```python
from build123d import *

# Parameters (mm, degrees)
SKIZZE1_W                       = 12
SKIZZE1_H                       = 17
AUFSATZ_LINEAR_AUSTRAGEN1_DEPTH = 2
SKIZZE3_W                       = 3
SKIZZE3_H                       = 1
SCHNITT_LINEAR_AUSTRAGEN1_DEPTH = 3
VERRUNDUNG1_R                   = 0.25


with BuildPart() as part:
    # Skizze1 → Aufsatz-Linear austragen1 (new body)
    with BuildSketch(Plane(origin=(0, 0, 0), x_dir=(1, 0, 0), z_dir=(0, 1, 0))):
        with Locations((6, 8.5)):
            Rectangle(SKIZZE1_W, SKIZZE1_H)
    extrude(amount=AUFSATZ_LINEAR_AUSTRAGEN1_DEPTH)

    # Skizze3 → Schnitt-Linear austragen1 (cut, through all)
    with BuildSketch(Plane(origin=(0, 2, 0), x_dir=(1, 0, 0), z_dir=(0, 1, 0))):
        with Locations((8.5, 2.5)):
            Rectangle(SKIZZE3_W, SKIZZE3_H)
        with Locations((3.5, 14.5)):
            Rectangle(SKIZZE3_W, SKIZZE3_H)
    extrude(amount=-SCHNITT_LINEAR_AUSTRAGEN1_DEPTH, mode=Mode.SUBTRACT)

    # Verrundung1
    verrundung1_edges = [part.edges().sort_by_distance(p)[0] for p in [
        (7, 1, -2),
        (10, 1, -2),
        (2, 1, -15),
        (5, 1, -15),
    ]]
    fillet(verrundung1_edges, radius=VERRUNDUNG1_R)


solid = part.part
```
Design review of the part built by this model. Coordinates are the model's own, in mm. A direction names the side the tool comes from. Coordinates: 2 decimals unless noted, no trailing zeros. Order: outer loops, then holes, each group sorted by start corner. A loop starts at its lowest first (then second) coordinate and runs counter-clockwise, first axis right, second up. Notation, with made-up numbers: (37.25, 19.25) - (72.25, 19.25) arc R25 cw to (72.25, 51.25) - close; hole circle Ø5 at (68.25, 18.25). An arc over 180 degrees is marked (long way). Answer in a Markdown table with one row per item.
(1) Clearance check with a flat-ended pin moving along its axis: pin 1 (1 mm diameter, centred on x = 3.5, y = 0.5, fed in from +Z). State where the tip first meets the part, or that it passes through.
Checked values:
| item | result |
|---|---|
| pin 1 | z = 0 |
(2) Consider section B-B on x = 9.5. State the section outline as (y, z) points, plus the area to 3 significant figures.
Checked values:
| item | result |
|---|---|
| outline | (0, -17) - (2, -17) - (2, -3) - (0, -3) - close; (0, -2) - (2, -2) - (2, 0) - (0, 0) - close |
| area | 32.0 mm^2 |
(3) The part is to be moulded in two halves that separate along X. For faces 3 (the flat face through (3, 1, -14)), 4 (the flat face through (6, 1, -17)), 5 (the flat face through (3, 1, -15)), 6 (the flat face through (0, 1, -8)), say which applies: released by +X, released by -X, zero draft, split by the parting line, or undercut.
Checked values:
| item | result |
|---|---|
| face 3 | undercut |
| face 4 | zero draft |
| face 5 | undercut |
| face 6 | released by -X |
(4) Consider section C-C on y = 0.2. State the section outline as (x, z) points.
Checked values:
| item | result |
|---|---|
| outline | (0, -17) - (12, -17) - (12, 0) - (0, 0) - close; hole (2, -14.75) arc R0.25 ccw to (2.25, -15) - (4.75, -15) arc R0.25 ccw to (5, -14.75) - (5, -14) - (2, -14) - close; hole (7, -3) - (10, -3) - (10, -2.25) arc R0.25 ccw to (9.75, -2) - (7.25, -2) arc R0.25 ccw to (7, -2.25) - close |
(5) Consider section A-A on z = -2.5. State the section outline as (x, y) points, plus the area to 3 significant figures.
Checked values:
| item | result |
|---|---|
| outline | (0, 0) - (7, 0) - (7, 2) - (0, 2) - close; (10, 0) - (12, 0) - (12, 2) - (10, 2) - close |
| area | 18.0 mm^2 |
(6) For faces 1 (the flat face through (6, 1, 0)), 2 (the flat face through (8, 1, -3)), list the 3-axis set-ups (+Z, -Z, +X, -X, +Y, -Y) from which the entire face can be reached by the end or side of a thin tool; tool diameter is ignored.
Checked values:
| item | result |
|---|---|
| face 1 | +Z, +X, -X, +Y, -Y |
| face 2 | +Y, -Y |
(7) Wall thickness on line 1 along Z through (x, y) = (3.75, 0.2); line 2 along Z through (x, y) = (8.75, 1): over which ranges is each line inside the solid? List them lowest first. Write a range as from..to.
Checked values:
| item | result |
|---|---|
| line 1 | -17..-15, -14..0 |
| line 2 | -17..-3, -2..0 |
